Input: part model. Units: mm. Frame: model coordinates. A direction names the side the tool comes from. Coordinates: 2 decimals unless noted, no trailing zeros. Write each loop counter-clockwise with the first axis right and the second up, starting at its lowest first coordinate (ties: lowest second). Pieces come first, ordered by that corner, then holes. Notation, with made-up numbers: (-17, 62) - (4, 62) arc R17 cw to (4, 68) - close; hole circle Ø2 at (12.25, -35). An arc over 180 degrees is marked (long way). Use a Markdown table: item, result. Add a question column.
Q1. Set-up query: faces 1 (the face through (-22.75, -0.08, 0.99)), 2 (the face through (-18.54, 1.44, 3.52)), 3 (the face through (-56, 1.5, 0)), 4 (the face through (-41, -3, -3)), 5 (the face through (-54, 0, -2)). Return all of +Z, -Z, +X, -X, +Y, -Y with unobstructed straight access to the full face (end or side cutting, diameter ignored); none if empty.
Q2. Section query D-D (x = -25.5). Return the cut outline in (y, z).
Q3. Section query B-B (x = -40.5). Return the cut outline in (y, z).
Q4. Material intervals for probe 1 along Z at (x, y) = (-57.75, -0.55); probe 2 along Y at (x, z) = (-34, -1.5); probe 3 along Y at (x, z) = (-21, 0.5), sorted ascending. Write a range as from..to.
Q5. Section query A-A (y = -1). Return the cut outline in (x, z), then the cut area to 3 significant figures.
Q6. Section query C-C (z = 3.25). Return the cut outline in (x, y).
Q7. Mould query, pull axis Z, two halves, no side actions, for faces 6 (the face through (-62.25, -0.06, 1.13)), 7 (the face through (-55.27, 3.021, 2.405)), 8 (the face through (-18.52, -1.405, 3.521)). Classes: released by +Z, released by -Z, zero draft, split by the parting line, or undercut.
Q8. Pin query (flat end, axial travel): P1, Ø1.7, axis at x = -22, y = -1.5, coming from the +Z side; P2, Ø4.5, axis at x = -20.5, y = 0.5, coming from the -Z side; P3, Ø0.9, axis at x = -58.5, y = 3, coming from the +Z side. Return the tip coordinate at first contact, or that it passes through.
Autodesk Inventor part; units mm, degrees
ref_plane "Płaszczyzna konstrukcyjna2" through (-16.0063, -4.5, 5) normal (0, 0, 1) x (1, 0, 0)
ref_plane "Płaszczyzna konstrukcyjna1" through (-25.5, -4.5, -3) normal (0, 0, -1) x (0, 1, 0)
ref_plane "YZ Plane" through (0, 0, 0) normal (1, 0, 0) x (0, 1, 0)
ref_plane "Płaszczyzna konstrukcyjna2" through (-16.0063, -4.5, 5) normal (0, 0, 1) x (1, 0, 0)
sketch "Szkic1" plane through (0, 0, 0) normal (0, 0, 1) x (1, 0, 0)
  circle A0 centre (-21, 0) radius 1.75
  arc A1 (-11.0125, 4.5) -> (-15.9781, 0.0856) centre (-11.0125, -0.5) ccw
  line L0 (-21, 4.5) -> (-11.0125, 4.5)
  arc A2 (-21, 4.5) -> (-21, -4.5) centre (-21, 0) ccw
  line L1 (-11.0628, -4.5) -> (-21, -4.5)
  arc A3 (-15.9446, -0.5811) -> (-11.0628, -4.5) centre (-11.0628, 0.5) ccw
  line L2 (-21, 0) -> (-57.75, 0)
  line L3 (-21, 0) -> (-57.75, 0) construction
  line L4 (-21, -4.5) -> (-57.75, -4.5)
  line L5 (-57.75, 4.5) -> (-21, 4.5)
  arc A4 (-21, -4.5) -> (-21, 4.5) centre (-21, 0) ccw
  arc A5 (-57.75, 4.5) -> (-57.75, -4.5) centre (-57.75, 0) ccw
  line L6 (-57.75, 4.5) -> (-57.75, -4.5)
  arc A6 (-15.9781, 0.0856) -> (-15.9446, -0.5811) centre (-13.9919, -0.1486) ccw
  point P0 (0, 0)
  point P1 (-39.375, 0)
  dimension "d0" = 36.75
extrude "Wyciągnięcie proste1" add sketch "Szkic1" along normal up to surface (5 mm away) contours A2 A4 | A2 L4 L6 L2 | L2 L6 L5 A2
sketch "Szkic2" plane through (0, 0, 0) normal (0, 0, -1) x (-1, 0, 0)
  line L0 (21, 4.5) -> (57.75, 4.5)
  arc A0 (21, 4.5) -> (21, -4.5) centre (21, 0) ccw
  line L1 (57.75, -4.5) -> (21, -4.5)
  line L2 (57.75, 4.5) -> (57.75, -4.5)
  circle A1 centre (21, 0) radius 1.75
  arc A2 (21, -4.5) -> (21, 4.5) centre (21, 0) ccw
  circle A3 centre (21, 0) radius 5
  point P0 (0, 0)
  point P1 (23.1794, 4.5)
  point P2 (23.1794, -4.5)
  dimension "d3" = 10
ref_plane "Płaszczyzna konstrukcyjna1" through (-25.5, -4.5, -3) normal (0, 0, -1) x (0, 1, 0)
extrude "Wyciągnięcie proste2" add sketch "Szkic2" along normal up to surface (3 mm away) contours L0 L2 L1 A3
fillet "Zaokrąglenie1" radius 4.5 2 edges at (-23.1794, -4.5, -1.5) (-23.1794, 4.5, -1.5)
sketch "Szkic4" plane through (-57.75, 4.5, 5) normal (0, 1, 0) x (1, 0, 0)
  line L0 (0, 8) -> (0, 0)
  circle A0 centre (0, 4) radius 1.75
  circle A1 centre (0, 4) radius 4
  point P0 (57.75, 5)
  point P1 (0, 2.25)
  point P2 (0, 5.75)
  dimension "d15" = 3.5
extrude "Wyciągnięcie proste6" add sketch "Szkic4" against normal up to surface (9 mm away) contours L0 A0 A1 picked at (-0.4587, 0.8057)
extrude "Wyciągnięcie proste7" cut sketch "Szkic4" against normal through all contours A0 L0 picked at (0.2531, 4.5256)
sketch "Szkic5" plane through (-30.5, 0, -3) normal (0, 0, -1) x (-1, 0, 0)
  arc A0 (0, 4.5) -> (0, -4.5) centre (0, 0) ccw
  line L0 (27.25, -4.5) -> (0, -4.5)
  line L1 (27.25, 4.5) -> (27.25, -4.5)
  line L2 (0, 4.5) -> (27.25, 4.5)
  line L3 (29, -4.5) -> (29, 4.5)
  line L4 (25.5, -4.5) -> (25.5, 4.5)
  line L5 (23.5, -4.5) -> (23.5, 4.5)
  arc A1 (0, 2.5) -> (0, -2.5) centre (0, 0) ccw
  line L6 (0, 2.5) -> (25.25, 2.5)
  line L7 (25.25, 2.5) -> (25.25, -2.5)
  line L8 (25.25, -2.5) -> (0, -2.5)
  point P0 (-30.5, 0)
  point P1 (23.5, -2.5)
  point P2 (23.5, 2.5)
  dimension "d20" = 2
  dimension "d21" = 2
extrude "Wyciągnięcie proste8" cut sketch "Szkic5" against normal up to surface (3 mm away) contours L5 L8 A1 L6
fillet "Zaokrąglenie2" radius 2 2 edges at (-54, 2.5, -1.5) (-54, -2.5, -1.5)
sketch "Szkic6" plane through (-21, 0, 5) normal (0, 0, 1) x (1, 0, 0)
  circle A0 centre (0, 0) radius 1.75
  circle A1 centre (0, 0) radius 2.85
  line L0 (1.6454, 2.85) -> (3.2909, 0)
  line L1 (3.2909, 0) -> (1.6454, -2.85)
  line L2 (1.6454, -2.85) -> (-1.6454, -2.85)
  line L3 (-1.6454, -2.85) -> (-3.2909, 0)
  line L4 (-3.2909, 0) -> (-1.6454, 2.85)
  line L5 (-1.6454, 2.85) -> (1.6454, 2.85)
  point P0 (21, 0)
  point P1 (0, 2.85)
  dimension "d25" = 5.7
extrude "Wyciągnięcie proste9" cut sketch "Szkic6" against normal blind 3 contours A0 | A1 | A1 L0 L1 | A1 L5 L0 | L1 L2 A1 | A1 L4 L5 | L2 L3 A1 | A1 L3 L4
sketch "Szkic7" plane through (-21, 4.5, 5) normal (0, 1, 0) x (1, 0, 0)
  circle A0 centre (-36.75, 4) radius 1.75
  circle A1 centre (-36.75, 4) radius 2.85
  circle A2 centre (-36.75, 4) radius 1.75
  line L0 (-35.1046, 6.85) -> (-33.4591, 4)
  line L1 (-33.4591, 4) -> (-35.1046, 1.15)
  line L2 (-35.1046, 1.15) -> (-38.3954, 1.15)
  line L3 (-38.3954, 1.15) -> (-40.0409, 4)
  line L4 (-40.0409, 4) -> (-38.3954, 6.85)
  line L5 (-38.3954, 6.85) -> (-35.1046, 6.85)
  point P0 (21, 5)
  point P1 (-36.75, 6.85)
  dimension "d28" = 5.7
extrude "Wyciągnięcie proste10" cut sketch "Szkic7" against normal blind 3 contours A0 | A1 | A1 L0 L1 | A1 L5 L0 | L1 L2 A1 | A1 L4 L5 | L2 L3 A1 | A1 L3 L4
sketch "Szkic8" plane through (-21, -4.5, 0) normal (0, -1, 0) x (1, 0, 0)
  circle A0 centre (-36.75, 1) radius 1.75
  circle A1 centre (-36.75, 1) radius 4.5
  arc A2 (-36.75, 5) -> (-36.75, -3) centre (-36.75, 1) ccw
  circle A3 centre (-36.75, 1) radius 1.75
  arc A4 (-36.75, 5) -> (-36.75, -3) centre (-36.75, 1) ccw
  line L0 (-36.75, -3) -> (-9.5, -3)
  line L1 (-9.5, 0) -> (-9.5, -3)
  line L2 (-9.5, 0) -> (0, 0)
  line L3 (0, 0) -> (0, 5)
  line L4 (0, 5) -> (-36.75, 5)
  point P0 (21, 0)
  point P1 (-34.6884, 5)
  point P2 (-34.6884, -3)
  dimension "d31" = 9
extrude "Wyciągnięcie proste11" add sketch "Szkic8" against normal up to surface (9 mm away) contours L4 A2 L0 A1 picked at (-35.7134, 5.1254)
properties part number "L1"
Values follow:
| question | item | result |
|---|---|---|
| 1 | face 1 | +Z, -Z |
| 1 | face 2 | +Z |
| 1 | face 3 | +Y |
| 1 | face 4 | -Z, +X, +Y, -Y |
| 1 | face 5 | -Z |
| 2 | outline | (-4.5, 0) - (4.5, 0) - (4.5, 5) - (-4.5, 5) - close |
| 3 | outline | (-4.5, -3) - (-2.5, -3) - (-2.5, 0) - (2.5, 0) - (2.5, -3) - (4.5, -3) - (4.5, 5) - (-4.5, 5) - close |
| 4 | probe 1 | -3.5..-0.75, 2.75..5.5 |
| 4 | probe 2 | -4.5..-2.5, 2.5..4.5 |
| 4 | probe 3 | -4.5..-1.75, 1.75..4.5 |
| 5 | outline | (-55.69, -3) - (-53.94, -3) - (-53.94, 0) - (-28.21, 0) - (-28.21, -3) - (-26.11, -3) - (-26.11, 0) - (-22.44, 0) - (-22.44, 2) - (-23.71, 2) - (-23.71, 5) - (-55.69, 5) arc R4.5 ccw (long way) to start; (-19.56, 0) - (-16.61, 0) - (-16.61, 5) - (-18.29, 5) - (-18.29, 2) - (-19.56, 2) - close; hole circle Ø3.5 at (-57.75, 1) |
| 5 | area | 225 mm2 |
| 6 | outline | (-61.65, -4.5) - (-21, -4.5) arc R4.5 ccw to (-21, 4.5) - (-55.76, 4.5) - (-55.76, 1.5) - (-59.74, 1.5) - (-59.74, 4.5) - (-61.65, 4.5) - close; hole (-24.29, 0) - (-22.65, -2.85) - (-19.35, -2.85) - (-17.71, 0) - (-19.35, 2.85) - (-22.65, 2.85) - close |
| 7 | face 6 | split by the parting line |
| 7 | face 7 | undercut |
| 7 | face 8 | zero draft |
| 8 | P1 | z = 2 |
| 8 | P2 | z = 0 |
| 8 | P3 | z = 5.49 |
